Work out the finished part from the listing and answer in its coordinate system (mm). Give positions to 0.01 mm unless a question says otherwise; leave off trailing zeros. Loops run counter-clockwise (first coordinate to the right, second up) from the corner with the lowest first, then second, coordinate; pieces in that order, holes last. Notation, with made-up numbers: (85, 14.25) - (107, 14.25) arc R15 cw to (107, 31.25) - close; hole circle Ø7 at (14.25, 33). An arc over 180 degrees is marked (long way). Use one line per item in the form item = value. Start each with the question number.
from build123d import *

# Parameters (mm, degrees)
ESBO_O1_R                  = 25.4
ESBO_O1_R_2                = 22.23
RESSALTO_EXTRUS_O1_DEPTH   = 300
CORTE_EXTRUS_O1_REACH      = 307.329
CORTE_EXTRUS_O1_END_RADIUS = 22.23
ESBO_O3_R                  = 2.5
PADR_OCIRCULAR1_COUNT      = 4
CORTE_EXTRUS_O2_REACH      = 307.329
CORTE_EXTRUS_O2_END_RADIUS = 22.23
ESBO_O4_R                  = 2.5
PADR_OCIRCULAR2_COUNT      = 4


with BuildPart() as part:
    # Esbo_o1 → Ressalto-extrus_o1 (new body)
    with BuildSketch(Plane.XY):
        Circle(ESBO_O1_R)
        Circle(ESBO_O1_R_2, mode=Mode.SUBTRACT)
    extrude(amount=RESSALTO_EXTRUS_O1_DEPTH)

    # Corte-extrus_o1: up to this cylinder (the profile starts outside it)
    corte_extrus_o1_end = Plane(origin=(0, 0, 292.5), z_dir=(0, 0, -1)) * Cylinder(CORTE_EXTRUS_O1_END_RADIUS, 660.118, mode=Mode.PRIVATE)
    # Esbo_o3 → Corte-extrus_o1 (cut, up to the surface)
    with BuildSketch(Plane(origin=(0, 25.4, 0), x_dir=(1, 0, 0), z_dir=(0, 1, 0)), mode=Mode.PRIVATE) as corte_extrus_o1_sk1:
        with Locations(Location((0, -292.5, 0), (0, 0, 270))):
            Circle(ESBO_O3_R)
    corte_extrus_o1_tool1 = extrude(corte_extrus_o1_sk1.sketch, amount=-CORTE_EXTRUS_O1_REACH, mode=Mode.PRIVATE) - corte_extrus_o1_end
    corte_extrus_o1 = corte_extrus_o1_tool1.solids().sort_by_distance((0, 25.4, 292.5))[0]
    add(corte_extrus_o1, mode=Mode.SUBTRACT)

    # Padr_oCircular1: Corte-extrus_o1 ×4 about axis
    padr_ocircular1_axis = Axis((0, 0, 300), (0, 0, 1))
    for i in range(1, PADR_OCIRCULAR1_COUNT):
        add(corte_extrus_o1.rotate(padr_ocircular1_axis, i * 360 / PADR_OCIRCULAR1_COUNT), mode=Mode.SUBTRACT)

    # Corte-extrus_o2: up to this cylinder (the profile starts outside it)
    corte_extrus_o2_end = Plane(origin=(0, 0, 7.5), z_dir=(0, 0, -1)) * Cylinder(CORTE_EXTRUS_O2_END_RADIUS, 660.118, mode=Mode.PRIVATE)
    # Esbo_o4 → Corte-extrus_o2 (cut, up to the surface)
    with BuildSketch(Plane(origin=(0, 25.4, 0), x_dir=(1, 0, 0), z_dir=(0, 1, 0)), mode=Mode.PRIVATE) as corte_extrus_o2_sk1:
        with Locations(Location((-0.017770346, -7.5, 0), (0, 0, 270))):
            Circle(ESBO_O4_R)
    corte_extrus_o2_tool1 = extrude(corte_extrus_o2_sk1.sketch, amount=-CORTE_EXTRUS_O2_REACH, mode=Mode.PRIVATE) - corte_extrus_o2_end
    corte_extrus_o2 = corte_extrus_o2_tool1.solids().sort_by_distance((-0.01777, 25.4, 7.5))[0]
    add(corte_extrus_o2, mode=Mode.SUBTRACT)

    # Padr_oCircular2: Corte-extrus_o2 ×4 about axis
    padr_ocircular2_axis = Axis((0, 0, 0), (0, 0, 1))
    for i in range(1, PADR_OCIRCULAR2_COUNT):
        add(corte_extrus_o2.rotate(padr_ocircular2_axis, i * 360 / PADR_OCIRCULAR2_COUNT), mode=Mode.SUBTRACT)


solid = part.part
1) Determine the mould class of faces 1 (the cylindrical face through (-23.77, -0.96, 294.81)), 2 (the cylindrical face through (-1, 23.8, 9.8)), 3 (the cylindrical face through (20.535, -8.514, 147.9)), 4 (the cylindrical face through (-5.506, -24.796, 147.9)) for opening direction X: released by +X, released by -X, zero draft, split by the parting line, or undercut.
2) A cutting plane is placed at D-D (z = 49). Give the vertices of the cut face in (x, y), plus the area to 3 significant figures.
3) Find the intervals of material crossed by probe 1 along Z at (x, y) = (0, -24); probe 2 along X at (y, z) = (1, 83); probe 3 along X at (y, z) = (-14.5, 14.5), in increasing order.
4) Flat-ended cylindrical pins translate along their axes: pin 1 Ø1.5 at (x, y) = (-19.5, 5) entering from -Z; pin 2 Ø2 at (x, z) = (-13, 76.5) entering from +Y; pin 3 Ø4 at (y, z) = (6.5, 60.5) entering from +X; pin 4 Ø3 at (x, z) = (-4, 246.5) entering from +Y. Find the tip coordinate at first contact, or state that the pin passes through.
5) A cutting plane is placed at A-A (y = 17.5). Give the vertices of the cut face in (x, z).
6) A cutting plane is placed at B-B (z = 292.5). Give the vertices of the cut face in (x, y).
7) A cutting plane is placed at C-C (x = -12). Give the vertices of the cut face in (y, z), plus the area to 3 significant figures.
Answer sheet:
q1.face_1 = zero draft
q1.face_2 = undercut
q1.face_3 = undercut
q1.face_4 = split by the parting line
q2.outline = circle Ø50.8 at (0, 0); hole circle Ø44.46 at (0, 0)
q2.area = 474 mm²
q3.probe_1 = 0 to 5, 10 to 290, 295 to 300
q3.probe_2 = -25.38 to -22.21, 22.21 to 25.38
q3.probe_3 = -20.85 to -16.85, 16.85 to 20.85
q4.pin_1 = through
q4.pin_2 = 22.39
q4.pin_3 = 25
q4.pin_4 = 25.28
q5.outline = (-18.41, 0) - (-13.71, 0) - (-13.71, 300) - (-18.41, 300) - close; (13.71, 0) - (18.41, 0) - (18.41, 300) - (13.71, 300) - close
q6.outline = (-25.28, -2.5) arc R25.4 ccw to (-2.5, -25.28) - (-2.5, -22.09) arc R22.23 cw to (-22.09, -2.5) - close; (-25.28, 2.5) - (-22.09, 2.5) arc R22.23 cw to (-2.5, 22.09) - (-2.5, 25.28) arc R25.4 ccw to start; (2.5, -25.28) arc R25.4 ccw to (25.28, -2.5) - (22.09, -2.5) arc R22.23 cw to (2.5, -22.09) - close; (2.5, 22.09) arc R22.23 cw to (22.09, 2.5) - (25.28, 2.5) arc R25.4 ccw to (2.5, 25.28) - close
q7.outline = (-22.39, 0) - (-18.71, 0) - (-18.71, 300) - (-22.39, 300) - close; (18.71, 0) - (22.39, 0) - (22.39, 300) - (18.71, 300) - close
q7.area = 2,200 mm²
